Source: CAD feature listing. Evaluate the final solid. Frame: model axes, mm. A direction names the side the tool comes from. Coordinates: 2 decimals unless noted, no trailing zeros. Write each loop counter-clockwise with the first axis right and the second up, starting at its lowest first coordinate (ties: lowest second). Pieces come first, ordered by that corner, then holes. Notation, with made-up numbers: (-18, 54.5) -> (37, 54.5) arc R8 ccw to (37, 63.5) -> close; hole circle Ø9 at (75.5, -4.5). An arc over 180 degrees is marked (long way). One line per item, written item: value. Start each with the question number.
1. First-contact query: P1, Ø1.5, axis at x = 1.5, y = -5.5, coming from the +Z side; P2, Ø1.6, axis at y = -13, z = 0.5, coming from the +X side; P3, Ø0.5, axis at y = -2.5, z = 4.5, coming from the -X side. Flat tips, straight axial feed; report the tip coordinate or a pass-through.
2. Section query A-A, the plane z = 3.45. Output: boundary loops of the cut face in (x, y), and give its area (3 significant figures).
3. Access query for faces 1 (the flat face through (-4, -16.737, 5)), 2 (the flat face through (8.22, -2.31, 2.73)), 3 (the flat face through (12, 3, 1)), 4 (the flat face through (3.4, -16.5, 0.7)). Directions: +Z, -Z, +X, -X, +Y, -Y. A direction counts if a zero-diameter tool reaches every point of the face in a straight line with its end or side. Return the directions, or none.
4. Section query B-B, the plane x = 1. Output: boundary loops of the cut face in (y, z), and give its area (3 significant figures).
5. Section query C-C, the plane y = -15. Output: boundary loops of the cut face in (x, z), and give its area (3 significant figures).
6. Line query: line 1 (Y direction, x = 0, z = 1.05); line 2 (Z direction, x = 2.5, y = -16.75); line 3 (X direction, y = -13.5, z = 0.3). Output: solid intervals per line, ascending.
7. Section query D-D, the plane x = 6.25. Output: boundary loops of the cut face in (y, z).
from build123d import *

# Parameters (mm, degrees)
EXTRUDE_1_DEPTH   = 6
EXTRUDE_1_2_DEPTH = 6
EXTRUDE_2_DEPTH   = 4
SKETCH_1_4_R      = 5
SKETCH_1_4_R_2    = 2.5
EXTRUDE_3_DEPTH   = 1.5


with BuildPart() as part:
    # Sketch 1 → Extrude 1 (new body)
    with BuildSketch(Plane.XY):
        Polygon((-3.5, -16.737022948), (-5, -16.737022948), (-5, -20), (1.73077212, -20), (1.73077212, -18.5), (-3.5, -18.5), align=None)
    extrude(amount=EXTRUDE_1_DEPTH)



with BuildPart() as body_2:
    # Sketch 1 → Extrude 1 2 (new body)
    with BuildSketch(Plane.XY):
        Polygon((15.25, 0.424756417), (11.995170544, -1.81504482), (11.995170544, -2.81504482), (16.5, 0.284940209), (16.5, 5.284940209), (15.25, 4.424756417), align=None)
    extrude(amount=EXTRUDE_1_2_DEPTH)


with BuildPart() as part_1:
    add(part.part)

    add(body_2.part)  # Extrude 2 merges body 2
    # Sketch 1_3 → Extrude 2 (add)
    with BuildSketch(Plane.XY):
        with BuildLine():
            ThreePointArc((-3.667720971, -3.398208775), (-4.655029799, -1.825019883), (-5, 0))
            Line((-5, 0), (-5, -16.737022948))
            Line((-5, -16.737022948), (-3.5, -16.737022948))
            Line((-3.5, -16.737022948), (-3.667720971, -3.398208775))
        make_face()
        with BuildLine():
            Line((1.73077212, -18.5), (1.73077212, -20))
            Line((1.73077212, -20), (3.012501912, -20))
            ThreePointArc((3.012501912, -20), (4.252676388, -19.536857224), (5.075756613, -18.5))
            Line((5.075756613, -18.5), (5.075756613, -17))
            ThreePointArc((5.075756613, -17), (4.268648237, -18.058826553), (3.012501912, -18.5))
            Line((3.012501912, -18.5), (1.73077212, -18.5))
        make_face()
        Polygon((14, 2.064572624), (12, 2.064572624), (11.995170544, -1.81504482), (15.25, 0.424756417), (15.25, 4.424756417), (14, 3.564572624), align=None)
        Polygon((8.372598905, -1.81504482), (8.063712244, -2.81504482), (11.995170544, -2.81504482), (11.995170544, -1.81504482), align=None)
    extrude(amount=EXTRUDE_2_DEPTH)

    # Sketch 1_4 → Extrude 3 (add)
    # profile 1 of 3: a face of its own
    with BuildSketch(Plane.XY):
        Circle(SKETCH_1_4_R)
        Circle(SKETCH_1_4_R_2, mode=Mode.SUBTRACT)
    # profile 2 of 3: a face of its own
    with BuildSketch(Plane.XY):
        with BuildLine():
            Line((1.360324879, 6.360324879), (0, 5))
            ThreePointArc((0, 5), (3.535533906, 3.535533906), (5, 0))
            ThreePointArc((5, 0), (4.778141361, -1.472876484), (4.132253945, -2.81504482))
            Line((4.132253945, -2.81504482), (8.063712244, -2.81504482))
            Line((8.063712244, -2.81504482), (8.372598905, -1.81504482))
            Line((8.372598905, -1.81504482), (11.995170544, -1.81504482))
            Line((11.995170544, -1.81504482), (12, 2.064572624))
            Line((12, 2.064572624), (12, 4.064572624))
            Line((12, 4.064572624), (1.360324879, 6.360324879))
        make_face()
    # profile 3 of 3: a face of its own
    with BuildSketch(Plane.XY):
        with BuildLine():
            ThreePointArc((1.73077212, -4.690887749), (-1.164344213, -4.862540751), (-3.667720971, -3.398208775))
            Line((-3.667720971, -3.398208775), (-3.5, -16.737022948))
            Line((-3.5, -16.737022948), (-3.5, -18.5))
            Line((-3.5, -18.5), (1.73077212, -18.5))
            Line((1.73077212, -18.5), (3.012501912, -18.5))
            ThreePointArc((3.012501912, -18.5), (4.268648237, -18.058826553), (5.075756613, -17))
            Line((5.075756613, -17), (1.73077212, -16))
            Line((1.73077212, -16), (1.73077212, -4.690887749))
        make_face()
    extrude(amount=EXTRUDE_3_DEPTH)


solid = part_1.part
Computed values:
1. P1: stops at z = 1.5
1. P2: stops at x = 1.73
1. P3: stops at x = 12
2. outline: (-5, -20) -> (3.01, -20) arc R2.47 ccw to (5.08, -18.5) -> (5.08, -17) arc R2.32 cw to (3.01, -18.5) -> (-3.5, -18.5) -> (-3.5, -16.74) -> (-3.67, -3.4) arc R5 cw to (-5, 0) -> close; (8.06, -2.82) -> (12, -2.82) -> (16.5, 0.28) -> (16.5, 5.28) -> (14, 3.56) -> (14, 2.06) -> (12, 2.06) -> (12, -1.82) -> (8.37, -1.82) -> close
2. area: 62.7 mm²
3. face 1: +Z, +X, -X, +Y
3. face 2: +Z, +Y
3. face 3: +Z, -Z, +Y
3. face 4: +Z, -Z, +X
4. outline: (-20, 0) -> (-2.29, 0) -> (-2.29, 1.5) -> (-18.5, 1.5) -> (-18.5, 6) -> (-20, 6) -> close; (2.29, 0) -> (6, 0) -> (6, 1.5) -> (2.29, 1.5) -> close
4. area: 38.9 mm²
5. outline: (-5, 0) -> (1.73, 0) -> (1.73, 1.5) -> (-3.52, 1.5) -> (-3.52, 4) -> (-5, 4) -> close
5. area: 13.8 mm²
6. line 1: y = -20 to -2.5, 2.5 to 5
6. line 2: z = 0 to 1.5
6. line 3: x = -5 to 1.73
7. outline: (-2.82, 0) -> (5.31, 0) -> (5.31, 1.5) -> (-2.82, 1.5) -> close
